```python
from build123d import *

# Parameters (mm, degrees)
EKSTR_ZYON_NCE1_DEPTH = 5
RADYUS1_R             = 0.5
IZIM2_R               = 1.5
KES_EKSTR_ZYON1_DEPTH = 10
IZIM4_R               = 1.5
KES_EKSTR_ZYON2_DEPTH = 10
SCALE3_SCALE          = 0.6


with BuildPart() as part:
    # Çizim1 → Ekstrüzyon-İnce1 (new, symmetric)
    with BuildSketch(Plane.XY):
        Polygon((20, 0), (0, 0), (0, 20), (-1, 20), (-1, -1), (20, -1), align=None)
    extrude(amount=EKSTR_ZYON_NCE1_DEPTH, both=True)

    # Radyus1
    radyus1_edges = [part.edges().sort_by_distance(p)[0] for p in [
        (-1, -1, 0),
        (0, 0, 0),
    ]]
    fillet(radyus1_edges, radius=RADYUS1_R)

    # Çizim2 → Kes-Ekstrüzyon1 (cut)
    with BuildSketch(Plane(origin=(0, 0, 0), x_dir=(0, 0, -1), z_dir=(1, 0, 0))):
        with Locations((0, 13)):
            Circle(IZIM2_R)
        with Locations((0, 5)):
            Circle(IZIM2_R)
    extrude(amount=-KES_EKSTR_ZYON1_DEPTH, mode=Mode.SUBTRACT)

    # Çizim4 → Kes-Ekstrüzyon2 (cut)
    with BuildSketch(Plane(origin=(0, 0, 0), x_dir=(1, 0, 0), z_dir=(0, 1, 0))):
        with Locations(Location((5, 0, 0), (0, 0, 270))):
            Circle(IZIM4_R)
        with Locations(Location((13, 0, 0), (0, 0, 270))):
            Circle(IZIM4_R)
    extrude(amount=-KES_EKSTR_ZYON2_DEPTH, mode=Mode.SUBTRACT)


with BuildPart() as part_1:
    # Scale3: scaled about (4.650907034, 4.650907034, 0)
    add(part.part.scale(SCALE3_SCALE).moved(Location((1.860362814, 1.860362814, 0))))


solid = part_1.part
```
Geometry check sheet. Reference: the model listing, model coordinates, mm. A direction names the side the tool comes from. Give positions to 0.01 mm unless a question says otherwise; leave off trailing zeros. Loops run counter-clockwise (first coordinate to the right, second up) from the corner with the lowest first, then second, coordinate; pieces in that order, holes last. Notation, with made-up numbers: M 61,69.25 L 106,69.25 A31 ccw 106,108.25 Z; hole C -36.75,-20 d8. An arc over 180 degrees is marked long. Write item = value, one per line. Start each with the question number.
1. Section check C-C, the plane z = -1.45. Enter the section's corners in (x, y).
2. Section check B-B, the plane x = 4.5. Enter the section's corners in (y, z).
3. Section check A-A, the plane z = 0. Enter the section's corners in (x, y).
4. Tool access check on faces 5 (the face through (1.86, 8, 0)), 6 (the face through (1.26, 8, 0)). Record the directions out of +Z, -Z, +X, -X, +Y, -Y that give a thin tool (end or side, any length) a straight path to the whole face; none if there is none.
5. Go/stop test with flat-tipped pins: P1, Ø1.1, axis at y = 9.66, z = 0, coming from the -X side; P2, Ø3, axis at x = 5.5, z = 1.5, coming from the +Y side; P3, Ø3, axis at y = 9, z = -0.5, coming from the +X side. Record where each tip stops, or that it passes through.
6. Draft check along Z on faces 1 (the face through (4.7, 1.5, -3)), 2 (the face through (3.982, 1.565, -0.195)), 3 (the face through (4.7, 1.5, 3)), 4 (the face through (1.565, 4.062, -0.415)). Enter one of: +Z half, -Z half, draft (parallel to the pull), parting line (faces both ways), or undercut.
7. Section check D-D, the plane y = 8. Enter the section's corners in (x, z), plus the area to 3 significant figures.
8. Thickness scan on probe 1 along Y at (x, z) = (1.7, 0); probe 2 along Y at (x, z) = (2.5, 1.75). Record the ranges inside material, lowest first.
Values follow:
q1.outline = M 1.26,1.56 A0.3 ccw 1.56,1.26 L 13.86,1.26 L 13.86,1.86 L 2.16,1.86 A0.3 cw 1.86,2.16 L 1.86,13.86 L 1.26,13.86 Z
q2.outline = M 1.26,-3 L 1.86,-3 L 1.86,-0.82 L 1.26,-0.82 Z; M 1.26,0.82 L 1.86,0.82 L 1.86,3 L 1.26,3 Z
q3.outline = M 1.26,1.56 A0.3 ccw 1.56,1.26 L 3.96,1.26 L 3.96,1.86 L 2.16,1.86 A0.3 cw 1.86,2.16 L 1.86,3.96 L 1.26,3.96 Z; M 1.26,5.76 L 1.86,5.76 L 1.86,8.76 L 1.26,8.76 Z; M 1.26,10.56 L 1.86,10.56 L 1.86,13.86 L 1.26,13.86 Z; M 5.76,1.26 L 8.76,1.26 L 8.76,1.86 L 5.76,1.86 Z; M 10.56,1.26 L 13.86,1.26 L 13.86,1.86 L 10.56,1.86 Z
q4.face_5 = +Z, -Z, +X, +Y
q4.face_6 = +Z, -Z, -X, +Y, -Y
q5.P1 = through
q5.P2 = 1.86
q5.P3 = 1.86
q6.face_1 = -Z half
q6.face_2 = undercut
q6.face_3 = +Z half
q6.face_4 = undercut
q7.outline = M 1.26,-3 L 1.86,-3 L 1.86,3 L 1.26,3 Z
q7.area = 3.60 mm^2
q8.probe_1 = 1.26 to 3.96, 5.76 to 8.76, 10.56 to 13.86
q8.probe_2 = 1.26 to 1.86
